The listing builds one solid part. Answer for the finished solid, in the listing's coordinates (mm). Face numbers are marked on the shaded views. Round coordinates to 2 decimals unless told otherwise and drop trailing zeros. Loops run counter-clockwise (first coordinate to the right, second up) from the corner with the lowest first, then second, coordinate; pieces in that order, holes last. Notation, with made-up numbers: (11, -5.5) -> (64, -5.5) arc R27 ccw to (64, 12.5) -> close; hole circle Ø9 at (26, 59.25). An arc over 180 degrees is marked (long way). Use a Markdown table: item, result. Add a question column.
Q1. For a pull along Z with two mould halves and no side action, classify the marked faces 1 and 2 as released by +Z, released by -Z, zero draft, split by the parting line, or undercut.
Q2. Section A-A on x = -8 is taken. Give the vertices of the cut face in (y, z).
Q3. Consider line 1 (Y direction, x = -96, z = 3.35); line 2 (Y direction, x = -77, z = 3.75); line 3 (Y direction, x = -97, z = 5.65). Determine where each line is inside the solid, lowest interval first.
Q4. Section C-C on z = 3.7 is taken. Give the number of separate pieces and of enclosed holes in the cut face, then the cut area to 3 significant figures.
Q5. Section B-B on y = 6 is taken. Give the vertices of the cut face in (x, z), then the cut area to 3 significant figures.
Q6. Section D-D on x = -45.5 is taken. Give the vertices of the cut face in (y, z).
Q7. Given pin 1 Ø2 at (y, z) = (30, 2.5) entering from +X; pin 2 Ø1.5 at (y, z) = (31.5, 3) entering from +X; pin 3 Ø3 at (x, z) = (-71.5, 2.5) entering from +Y, each flat-ended and moving along its own axis, determine where each tip first touches the part or whether it passes through.
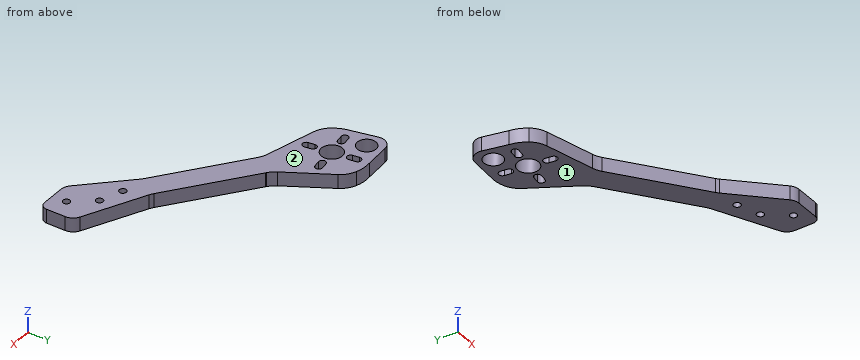
from build123d import *

# Parameters (mm, degrees)
CROQUIS1_R              = 1.5
CROQUIS1_R_2            = 4
CROQUIS1_R_3            = 4.5
SALIENTE_EXTRUIR1_DEPTH = 6


with BuildPart() as part:
    # Croquis1 → Saliente-Extruir1 (new body)
    with BuildSketch(Plane.XY):
        with BuildLine():
            Line((0, 3), (0, 11.005922656))
            ThreePointArc((0, 11.005922656), (-0.772770469, 13.676227974), (-2.852212196, 15.521120055))
            Line((-2.852212196, 15.521120055), (-28.127681877, 27.544148224))
            ThreePointArc((-28.127681877, 27.544148224), (-29.001474549, 28.014307534), (-29.824371512, 28.568747792))
            Line((-29.824371512, 28.568747792), (-63.171065255, 53.528446126))
            Line((-63.171065255, 53.528446126), (-63.451967787, 53.738699128))
            ThreePointArc((-63.451967787, 53.738699128), (-64.905667664, 55.069346162), (-66.070176318, 56.659246931))
            Line((-66.070176318, 56.659246931), (-76.965636536, 75.10772477))
            ThreePointArc((-76.965636536, 75.10772477), (-79.204988458, 77.730188181), (-82.201994916, 79.436049742))
            ThreePointArc((-82.201994916, 79.436049742), (-85.75594879, 80.239775378), (-89.398839068, 80.162876369))
            Line((-89.398839068, 80.162876369), (-99.846657066, 79.479321846))
            ThreePointArc((-99.846657066, 79.479321846), (-103.523124692, 77.4861215), (-104.39928334, 73.396915238))
            Line((-104.39928334, 73.396915238), (-102.110353231, 63.180020081))
            ThreePointArc((-102.110353231, 63.180020081), (-101.157367153, 59.663149232), (-99.384526804, 56.479817622))
            ThreePointArc((-99.384526804, 56.479817622), (-96.903104349, 54.085124746), (-93.75579069, 52.675717741))
            Line((-93.75579069, 52.675717741), (-72.984328521, 47.421790897))
            ThreePointArc((-72.984328521, 47.421790897), (-71.130664391, 46.752616664), (-69.44423303, 45.732903898))
            Line((-69.44423303, 45.732903898), (-35.612091664, 20.409852413))
            ThreePointArc((-35.612091664, 20.409852413), (-35.03729077, 19.945518736), (-34.498346176, 19.44000854))
            Line((-34.498346176, 19.44000854), (-16.717412791, 1.482024321))
            ThreePointArc((-16.717412791, 1.482024321), (-15.089260875, 0.385356005), (-13.164407425, 0))
            Line((-13.164407425, 0), (-3, 0))
            ThreePointArc((-3, 0), (-0.878679656, 0.878679656), (0, 3))
        make_face()
        with Locations((-24.85, 18.6)):
            Circle(CROQUIS1_R, mode=Mode.SUBTRACT)
        with Locations((-8, 6)):
            Circle(CROQUIS1_R, mode=Mode.SUBTRACT)
        with Locations((-97.670701805, 73.105635959)):
            Circle(CROQUIS1_R_2, mode=Mode.SUBTRACT)
        with Locations((-87.263168006, 65.315691143)):
            Circle(CROQUIS1_R_3, mode=Mode.SUBTRACT)
        with Locations((-15.25, 15.25)):
            Circle(CROQUIS1_R, mode=Mode.SUBTRACT)
        with BuildLine():
            Line((-87.237824709, 75.67483482), (-86.839166111, 72.903360245))
            ThreePointArc((-86.839166111, 72.903360245), (-88.110317527, 71.205074616), (-89.808603156, 72.476226032))
            Line((-89.808603156, 72.476226032), (-90.207261755, 75.247700608))
            ThreePointArc((-90.207261755, 75.247700608), (-88.936110338, 76.945986237), (-87.237824709, 75.67483482))
        make_face(mode=Mode.SUBTRACT)
        with BuildLine():
            Line((-76.904024329, 65.290347847), (-79.675498905, 64.891689248))
            ThreePointArc((-79.675498905, 64.891689248), (-81.373784533, 66.162840665), (-80.102633117, 67.861126294))
            Line((-80.102633117, 67.861126294), (-77.331158542, 68.259784892))
            ThreePointArc((-77.331158542, 68.259784892), (-75.632872913, 66.988633476), (-76.904024329, 65.290347847))
        make_face(mode=Mode.SUBTRACT)
        with BuildLine():
            Line((-87.288511303, 54.956547467), (-87.687169901, 57.728022042))
            ThreePointArc((-87.687169901, 57.728022042), (-86.416018485, 59.426307671), (-84.717732856, 58.155156254))
            Line((-84.717732856, 58.155156254), (-84.319074258, 55.383681679))
            ThreePointArc((-84.319074258, 55.383681679), (-85.590225674, 53.68539605), (-87.288511303, 54.956547467))
        make_face(mode=Mode.SUBTRACT)
        with BuildLine():
            Line((-97.622311683, 65.34103444), (-94.850837108, 65.739693038))
            ThreePointArc((-94.850837108, 65.739693038), (-93.152551479, 64.468541622), (-94.423702895, 62.770255993))
            Line((-94.423702895, 62.770255993), (-97.19517747, 62.371597395))
            ThreePointArc((-97.19517747, 62.371597395), (-98.893463099, 63.642748811), (-97.622311683, 65.34103444))
        make_face(mode=Mode.SUBTRACT)
    extrude(amount=SALIENTE_EXTRUIR1_DEPTH)


solid = part.part
Checked values:
| question | item | result |
|---|---|---|
| 1 | face 1 | released by -Z |
| 1 | face 2 | released by +Z |
| 2 | outline | (0, 0) -> (4.5, 0) -> (4.5, 6) -> (0, 6) -> close; (7.5, 0) -> (17.97, 0) -> (17.97, 6) -> (7.5, 6) -> close |
| 3 | line 1 | y = 53.54 to 62.54, 65.57 to 69.47, 76.74 to 79.73 |
| 3 | line 2 | y = 48.44 to 65.28, 68.27 to 75.17 |
| 3 | line 3 | y = 54.15 to 62.4, 65.43 to 69.16, 77.05 to 79.67 |
| 4 | separate pieces | 1 |
| 4 | enclosed holes | 9 |
| 4 | area | 1,700 mm2 |
| 5 | outline | (-21.19, 0) -> (-9.5, 0) -> (-9.5, 6) -> (-21.19, 6) -> close; (-6.5, 0) -> (0, 0) -> (0, 6) -> (-6.5, 6) -> close |
| 5 | area | 109 mm2 |
| 6 | outline | (27.81, 0) -> (40.3, 0) -> (40.3, 6) -> (27.81, 6) -> close |
| 7 | pin 1 | stops at x = -30.4 |
| 7 | pin 2 | stops at x = -32.74 |
| 7 | pin 3 | stops at y = 68.39 |
